```python
from build123d import *

# Parameters (mm, degrees)
PAD_DEPTH       = 47
SKETCH001_R     = 11
PAD001_DEPTH    = 2
SKETCH002_R     = 2.5
PAD002_DEPTH    = 22
SKETCH003_W     = 1
SKETCH003_H     = 4
POCKET_DEPTH    = 21
SKETCH004_R     = 1.5
POCKET001_DEPTH = 4.5


with BuildPart() as part:
    # Sketch → Pad (new body)
    with BuildSketch(Plane.XY):
        with BuildLine():
            Line((-16.65, -21.15), (16.65, -21.15))
            ThreePointArc((16.65, -21.15), (19.033457, -19.033457), (21.15, -16.65))
            Line((21.15, -16.65), (21.15, 16.65))
            ThreePointArc((21.15, 16.65), (19.033457, 19.033457), (16.65, 21.15))
            Line((16.65, 21.15), (-16.65, 21.15))
            ThreePointArc((-16.65, 21.15), (-19.033457, 19.033457), (-21.15, 16.65))
            Line((-21.15, 16.65), (-21.15, -16.65))
            ThreePointArc((-21.15, -16.65), (-19.033457, -19.033457), (-16.65, -21.15))
        make_face()
    extrude(amount=PAD_DEPTH)

    # Sketch001 → Pad001 (new body)
    with BuildSketch(Plane.XY.offset(47)):
        Circle(SKETCH001_R)
    extrude(amount=PAD001_DEPTH)

    # Sketch002 → Pad002 (new body)
    with BuildSketch(Plane.XY.offset(49)):
        Circle(SKETCH002_R)
    extrude(amount=PAD002_DEPTH)

    # Sketch003 → Pocket (cut)
    with BuildSketch(Plane.XY.offset(71)):
        with Locations((2.5, 0)):
            Rectangle(SKETCH003_W, SKETCH003_H)
    extrude(amount=-POCKET_DEPTH, mode=Mode.SUBTRACT)

    # Sketch004 → Pocket001 (cut)
    with BuildSketch(Plane.XY.offset(47)):
        with Locations((-15.5, 15.5)):
            Circle(SKETCH004_R)
        with Locations((15.5, 15.5)):
            Circle(SKETCH004_R)
        with Locations((-15.5, -15.5)):
            Circle(SKETCH004_R)
        with Locations((15.5, -15.5)):
            Circle(SKETCH004_R)
    extrude(amount=-POCKET001_DEPTH, mode=Mode.SUBTRACT)


solid = part.part
```
For this review, take the finished solid that the model builds, in its own axes (mm). A direction names the side the tool comes from. Coordinates: 2 decimals unless noted, no trailing zeros. Order: outer loops, then holes, each group sorted by start corner. A loop starts at its lowest first (then second) coordinate and runs counter-clockwise, first axis right, second up. Notation, with made-up numbers: (79, 73.25) - (135, 73.25) arc R13 cw to (135, 85.25) - close; hole circle Ø3 at (59, -26.75). An arc over 180 degrees is marked (long way). Answer as a JSON object with one key per item and string values. Group by question number.
1. We need section A-A on x = 0. State the section outline as (y, z) points, then the cut area to 3 significant figures.
2. Clearance check with flat-ended pins moving along their axes: P1, Ø0.9, axis at y = 0.5, z = 61, coming from the +X side; P2, Ø3.5, axis at x = -15, y = 15.5, coming from the +Z side; P3, Ø6.5, axis at x = 4, y = 3, coming from the +Z side; P4, Ø1.8, axis at x = -15.5, y = 15.5, coming from the +Z side. State where each tip first meets the part, or that it passes through.
3. We need section D-D on y = 15.5. State the section outline as (x, z) points, then the cut area to 3 significant figures.
4. For probe 1 along Y at (x, z) = (15.5, 44.8); probe 2 along Y at (x, z) = (15, 44), list the stretches that pass through material, from the lowest coordinate up.
5. The part is to be moulded in two halves that separate along X. For faces 4 (the cylindrical face through (19.002, -19.065, 23.171)), 5 (the cylindrical face through (-19.002, 19.065, 23.171)), 6 (the cylindrical face through (14, 15.57, 44.78)), say which applies: pulls with the +X half, pulls with the -X half, needs draft (parallel to the pull), parting line crosses it, or undercut.
6. We need section C-C on z = 21. State the section outline as (x, y) points, then the cut area to 3 significant figures.
7. We need section B-B on y = 0. State the section outline as (x, z) points.
8. For faces 1 (the flat face through (2, 0, 61)), 2 (the flat face through (0, 0, 71)), 3 (the cylindrical face through (-2.38, -10.74, 47.99)), list the 3-axis set-ups (+Z, -Z, +X, -X, +Y, -Y) from which the entire face can be reached by the end or side of a thin tool; tool diameter is ignored.
Final values:
{
 "1": {"outline": "(-21.15, 0) - (21.15, 0) - (21.15, 47) - (11, 47) - (11, 49) - (2.5, 49) - (2.5, 71) - (-2.5, 71) - (-2.5, 49) - (-11, 49) - (-11, 47) - (-21.15, 47) - close", "area": "2,140 mm²"},
 "2": {"P1": "x = 2", "P2": "z = 47", "P3": "z = 71", "P4": "z = 42.5"},
 "3": {"outline": "(-21.15, 0) - (21.15, 0) - (21.15, 47) - (17, 47) - (17, 42.5) - (14, 42.5) - (14, 47) - (-14, 47) - (-14, 42.5) - (-17, 42.5) - (-17, 47) - (-21.15, 47) - close", "area": "1,960 mm²"},
 "4": {"probe 1": "-21.15 to -17, -14 to 14, 17 to 21.15", "probe 2": "-21.15 to -16.91, -14.09 to 14.09, 16.91 to 21.15"},
 "5": {"face 4": "pulls with the +X half", "face 5": "pulls with the -X half", "face 6": "undercut"},
 "6": {"outline": "(-21.15, -16.65) arc R26.92 ccw to (-16.65, -21.15) - (16.65, -21.15) arc R26.92 ccw to (21.15, -16.65) - (21.15, 16.65) arc R26.92 ccw to (16.65, 21.15) - (-16.65, 21.15) arc R26.92 ccw to (-21.15, 16.65) - close", "area": "1,750 mm²"},
 "7": {"outline": "(-21.15, 0) - (21.15, 0) - (21.15, 47) - (11, 47) - (11, 49) - (2.5, 49) - (2.5, 50) - (2, 50) - (2, 71) - (-2.5, 71) - (-2.5, 49) - (-11, 49) - (-11, 47) - (-21.15, 47) - close"},
 "8": {"face 1": "+Z, +X, +Y, -Y", "face 2": "+Z, +X, -X, +Y, -Y", "face 3": "+Z"}
}
